Check sheet for the modelled part. Datum: model origin and axes. Units: mm. Coordinates: 2 decimals unless noted, no trailing zeros. Write each loop counter-clockwise with the first axis right and the second up, starting at its lowest first coordinate (ties: lowest second). Pieces come first, ordered by that corner, then holes. Notation, with made-up numbers: M 67,-32 L 120,-32 A20 cw 120,-16 Z; hole C 32,46 d6. An arc over 180 degrees is marked long. Answer as CSV lines item,"result". Start each with the question number.
1) Section check B-B (y = -54.5). Record the cut outline in (x, z).
2) Section check C-C (z = 79). Record the cut outline in (x, y), and give its area (3 significant figures).
3) Go/stop test with flat-tipped pins: pin 1 Ø2 at (x, y) = (2, -51.5) entering from +Z; pin 2 Ø1.7 at (x, z) = (1, 12.5) entering from -Y; pin 3 Ø4.5 at (y, z) = (0, 0) entering from +X (3 decimals); pin 4 Ø2 at (x, y) = (0.5, -31.5) entering from +Z. Record where each tip stops, or that it passes through.
4) Material ranges on L1, parallel to Y at x = 1.6, z = 31; L2, parallel to Z at x = 0.95, y = 0; L3, parallel to Z at x = -0.25, y = 1, recorded low to high. Write a range as [from, to].
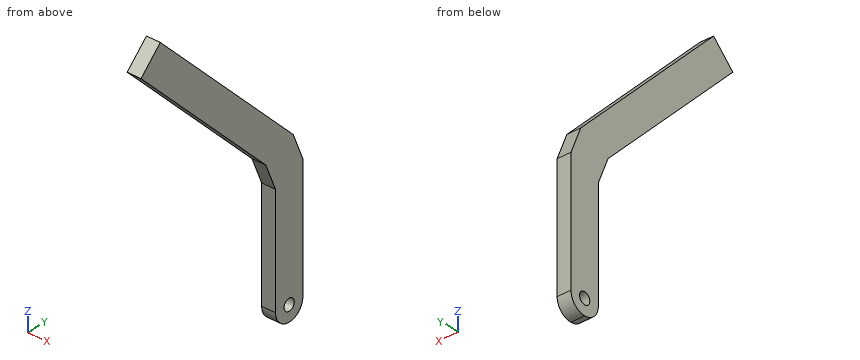
from build123d import *

# Parameters (mm, degrees)
F1_DEPTH = 2.8575
F3_D     = 4.7625
F4_R     = 6.34999
F5_SIZE  = 6.35


# Not quite as in the source:
# - a fillet or chamfer is up to 0.001 mm smaller than in the source, because OpenCascade refuses the exact size


with BuildPart() as f1:
    # F0 (on Right) → F1 (new body, symmetric)
    with BuildSketch(Plane.YZ):
        Polygon((6.35, -6.35), (6.35, 56.3145122421), (-59.8537438789, 122.5182561211), (-68.834, 113.538), (-6.35, 51.054), (-6.35, -6.35), align=None)
    extrude(amount=F1_DEPTH, both=True)

    # F3 (through all)
    with Locations(Plane.YZ.offset(2.8575)):
        with Locations((0, 0)):
            Hole(F3_D / 2)

    # F4 (radius 6.35 in the source; OpenCascade refuses exactly that, so slightly less here)
    f4_edges = [f1.edges().sort_by_distance(p)[0] for p in [
        (0, -6.35, -6.35),
        (0, 6.35, -6.35),
    ]]
    fillet(f4_edges, radius=F4_R)

    # F5
    f5_edges = [f1.edges().sort_by_distance(p)[0] for p in [
        (0, -6.35, 51.054),
        (0, 6.35, 56.314512),
    ]]
    chamfer(f5_edges, length=F5_SIZE)


solid = f1.part
Results found:
1,outline,"M -2.86,99.2 L 2.86,99.2 L 2.86,117.16 L -2.86,117.16 Z"
2,outline,"M -2.86,-34.3 L 2.86,-34.3 L 2.86,-16.34 L -2.86,-16.34 Z"
2,area,"103 mm2"
3,pin 1,"stops at z = 115.16"
3,pin 2,"stops at y = -6.35"
3,pin 3,"passes through"
3,pin 4,"stops at z = 95.16"
4,L1,"y = [-6.35, 6.35]"
4,L2,"z = [-6.35, -2.38], [2.38, 62.66]"
4,L3,"z = [-6.27, -2.16], [2.16, 61.66]"
